from build123d import *

# Parameters (mm, degrees)
F1_DEPTH = 12.7


with BuildPart() as f1:
    # F0 (on Top) → F1 (new body)
    with BuildSketch(Plane.XY):
        with BuildLine():
            Line((7.714299, 0), (0, 0))
            Line((0, 0), (-7.714299, 0))
            Line((-7.714299, 0), (-8.022307, 9.800587))
            Line((-8.022307, 9.800587), (-13.498154, -6.533614))
            ThreePointArc((-13.498154, -6.533614), (-20.995744, -7.940171), (-28.493334, -6.533614))
            ThreePointArc((-28.493334, -6.533614), (-31.465941, 5.890964), (-28.493334, 18.315542))
            ThreePointArc((-28.493334, 18.315542), (-57.349967, -11.034002), (-48.843939, -51.30494))
            ThreePointArc((-48.843939, -51.30494), (-47.885852, -38.32362), (-38.775746, -29.026385))
            ThreePointArc((-38.775746, -29.026385), (-33.628454, -29.072653), (-29.987374, -32.711237))
            ThreePointArc((-29.987374, -32.711237), (-27.56038, -27.988323), (-22.399301, -26.739529))
            ThreePointArc((-22.399301, -26.739529), (-18.405939, -28.296448), (-17.654907, -32.516268))
            ThreePointArc((-17.654907, -32.516268), (-14.956693, -29.974504), (-11.249818, -29.972308))
            ThreePointArc((-11.249818, -29.972308), (-4.691706, -37.79257), (0, -46.85641))
            ThreePointArc((0, -46.85641), (4.691706, -37.79257), (11.249818, -29.972308))
            ThreePointArc((11.249818, -29.972308), (14.956693, -29.974504), (17.654907, -32.516268))
            ThreePointArc((17.654907, -32.516268), (18.405939, -28.296448), (22.399301, -26.739529))
            ThreePointArc((22.399301, -26.739529), (27.56038, -27.988323), (29.987374, -32.711237))
            ThreePointArc((29.987374, -32.711237), (33.628454, -29.072653), (38.775746, -29.026385))
            ThreePointArc((38.775746, -29.026385), (47.885852, -38.32362), (48.843939, -51.30494))
            ThreePointArc((48.843939, -51.30494), (57.349967, -11.034002), (28.493334, 18.315542))
            ThreePointArc((28.493334, 18.315542), (31.465941, 5.890964), (28.493334, -6.533614))
            ThreePointArc((28.493334, -6.533614), (20.995744, -7.940171), (13.498154, -6.533614))
            Line((13.498154, -6.533614), (8.022307, 9.800587))
            Line((8.022307, 9.800587), (7.714299, 0))
        make_face()
    extrude(amount=F1_DEPTH)


solid = f1.part
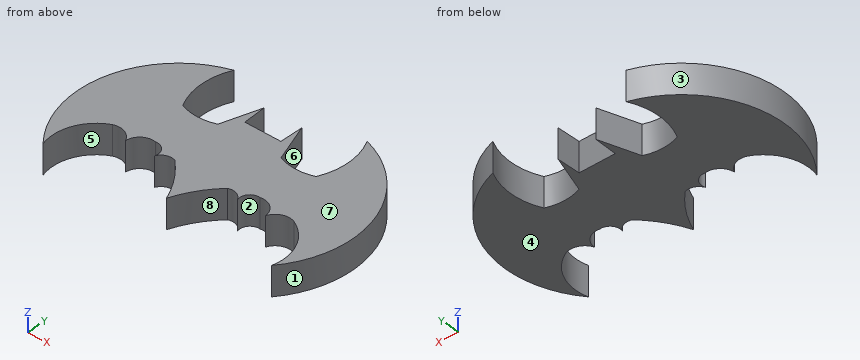
Part model, mm, in its own coordinate system. Face numbers are marked on the shaded views. A direction names the side the tool comes from. Coordinates: 2 decimals unless noted, no trailing zeros. Order: outer loops, then holes, each group sorted by start corner. A loop starts at its lowest first (then second) coordinate and runs counter-clockwise, first axis right, second up.
(1) Slice it at B-B, the plane y = 8. Write the cut outline in (x, z).
Check sheet entries:
outline: (-45.87, 0) - (-31.38, 0) - (-31.38, 12.7) - (-45.87, 12.7) - close; (-8.63, 0) - (-7.97, 0) - (-7.97, 12.7) - (-8.63, 12.7) - close; (7.97, 0) - (8.63, 0) - (8.63, 12.7) - (7.97, 12.7) - close; (31.38, 0) - (45.87, 0) - (45.87, 12.7) - (31.38, 12.7) - close
(2) Slice it at C-C, the plane z = 2.5. Write the cut outline in (x, y), and give its area (3 significant figures).
Check sheet entries:
outline: (-48.84, -51.3) arc R18.94 cw to (-38.78, -29.03) arc R6.8 cw to (-29.99, -32.71) arc R6.38 cw to (-22.4, -26.74) arc R4.38 cw to (-17.65, -32.52) arc R5.03 cw to (-11.25, -29.97) arc R46.45 cw to (0, -46.86) arc R46.45 cw to (11.25, -29.97) arc R5.03 cw to (17.65, -32.52) arc R4.38 cw to (22.4, -26.74) arc R6.38 cw to (29.99, -32.71) arc R6.8 cw to (38.78, -29.03) arc R18.94 cw to (48.84, -51.3) arc R43.52 ccw to (28.49, 18.32) arc R27.45 cw to (28.49, -6.53) arc R20.69 cw to (13.5, -6.53) - (8.02, 9.8) - (7.71, 0) - (-7.71, 0) - (-8.02, 9.8) - (-13.5, -6.53) arc R20.69 cw to (-28.49, -6.53) arc R27.45 cw to (-28.49, 18.32) arc R43.52 ccw to start
area: 4,090 mm2
(3) Pull direction X, two halves, no side cores. Call the marked faces 1, 2 and 3: pulls with the +X half, pulls with the -X half, needs draft (parallel to the pull), parting line crosses it, or undercut.
Check sheet entries:
face 1: pulls with the +X half
face 2: undercut
face 3: pulls with the -X half
(4) Pin check, flat tips, straight feed: pin 1 Ø6 at (x, z) = (4.5, 11) entering from +Y; pin 2 Ø4 at (x, z) = (-46, 9) entering from -Y; pin 3 Ø4 at (y, z) = (-10.5, 4.5) entering from +X. Stop position of each tip, or through.
Check sheet entries:
pin 1: stops at y = 0
pin 2: stops at y = -38.58
pin 3: stops at x = 57.75
(5) Probe L1, parallel to X at y = 3, z = 12.25; L2, parallel to X at y = 8.5, z = 5.5; L3, parallel to X at y = -44.5, z = 2.25. List the from-to ranges inside material, lowest first.
Check sheet entries:
L1: x = -50.29 to -31.31, -10.3 to -7.81, 7.81 to 10.3, 31.31 to 50.29
L2: x = -45.35 to -31.34, -8.46 to -7.98, 7.98 to 8.46, 31.34 to 45.35
L3: x = -53.55 to -49.5, -0.98 to 0.98, 49.5 to 53.55
(6) Slice it at A-A, the plane y = -4.5. Write the cut outline in (x, z), and give its area (3 significant figures).
Check sheet entries:
outline: (-54.85, 0) - (-29.42, 0) - (-29.42, 12.7) - (-54.85, 12.7) - close; (-12.82, 0) - (12.82, 0) - (12.82, 12.7) - (-12.82, 12.7) - close; (29.42, 0) - (54.85, 0) - (54.85, 12.7) - (29.42, 12.7) - close
area: 971 mm2
(7) Tool access for the marked faces 4, 5, 6, 7 and 8: list every direction of +Z, -Z, +X, -X, +Y, -Y with a clear straight run to the whole face (end or side of a thin tool).
Check sheet entries:
face 4: -Z, +X, -X, +Y, -Y
face 5: +Z, -Z
face 6: +Z, -Z, +Y
face 7: +Z, +X, -X, +Y, -Y
face 8: +Z, -Z, -Y
(8) Slice it at D-D, the plane y = -39.5. Write the cut outline in (x, z).
Check sheet entries:
outline: (-55.95, 0) - (-48.37, 0) - (-48.37, 12.7) - (-55.95, 12.7) - close; (-3.61, 0) - (3.61, 0) - (3.61, 12.7) - (-3.61, 12.7) - close; (48.37, 0) - (55.95, 0) - (55.95, 12.7) - (48.37, 12.7) - close
